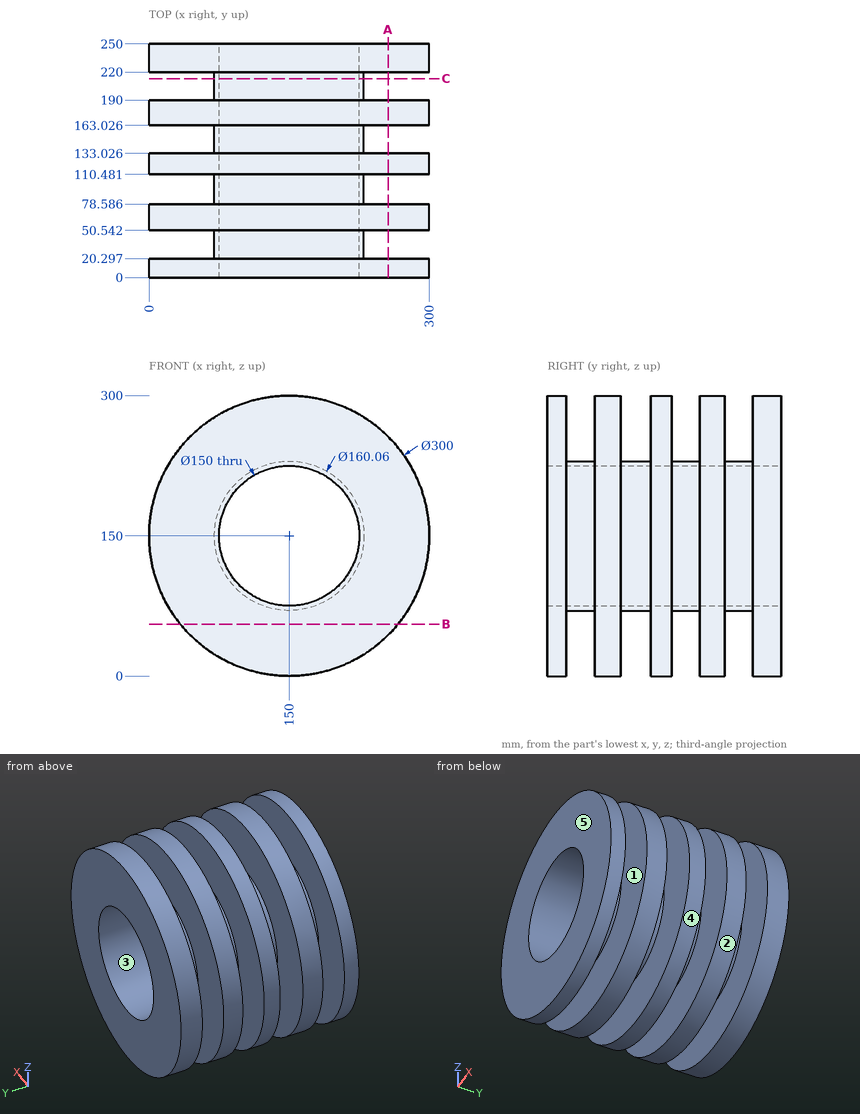
Source: three-view drawing plus pictorial views. Frame: mm from the lowest corner of the part. A direction names the side the tool comes from. Round coordinates to 2 decimals unless told otherwise and drop trailing zeros. Write each loop counter-clockwise with the first axis right and the second up, starting at its lowest first coordinate (ties: lowest second). Pieces come first, ordered by that corner, then holes. Notation, with made-up numbers: M 70,49.25 L 88,49.25 A6 cw 88,54.25 Z; hole C 71,54 d4. An arc over 180 degrees is marked long. One line per item, written item: value. Start each with the question number.
Item 1: Section query A-A (x = 256). Return the cut outline in (y, z).
Item 2: Section query C-C (y = 213). Return the cut outline in (x, z), plus the area to 3 significant figures.
Item 3: Set-up query: the marked faces 1 and 2. Return all of +Z, -Z, +X, -X, +Y, -Y with unobstructed straight access to the full face (end or side cutting, diameter ignored); none if empty.
Item 4: Mould query, pull axis Z, two halves, no side actions, for the marked faces 3, 4 and 5. Classes: pulls with the +Z half, pulls with the -Z half, needs draft (parallel to the pull), parting line crosses it, or undercut.
Item 5: Ray query, L1, parallel to Y at x = 188, z = 50; L2, parallel to X at y = 160.5, z = 150; L3, parallel to X at y = 62, z = 150. Return the intervals inside material, ascending. Write a range as from..to.
Item 6: Section query B-B (z = 55.5). Return the cut outline in (x, y).
Item 7: Pin query (flat end, axial travel): pin 1 (10 mm diameter, centred on y = 43.5, z = 195, fed in from -X); pin 2 (10 mm diameter, centred on y = 25, z = 208, fed in from +X); pin 3 (4 mm diameter, centred on y = 45, z = 214, fed in from -X) (1 decimal). Return the tip coordinate at first contact, or that it passes through.
Result set:
1. outline: M 0,43.87 L 20.3,43.87 L 20.3,256.13 L 0,256.13 Z; M 50.54,43.87 L 78.59,43.87 L 78.59,256.13 L 50.54,256.13 Z; M 110.48,43.87 L 133.03,43.87 L 133.03,256.13 L 110.48,256.13 Z; M 163.03,43.87 L 190,43.87 L 190,256.13 L 163.03,256.13 Z; M 220,43.87 L 250,43.87 L 250,256.13 L 220,256.13 Z
2. outline: C 150,150 d160.06; hole C 150,150 d150
2. area: 2,450 mm²
3. face 1: none
3. face 2: +Y, -Y
4. face 3: undercut
4. face 4: parting line crosses it
4. face 5: needs draft
5. L1: y = 0..20.3, 50.54..78.59, 110.48..133.03, 163.03..190, 220..250
5. L2: x = 69.97..75, 225..230.03
5. L3: x = 0..75, 225..300
6. outline: M 33.51,0 L 266.49,0 L 266.49,20.3 L 33.51,20.3 Z; M 33.51,50.54 L 266.49,50.54 L 266.49,78.59 L 33.51,78.59 Z; M 33.51,110.48 L 266.49,110.48 L 266.49,133.03 L 33.51,133.03 Z; M 33.51,163.03 L 266.49,163.03 L 266.49,190 L 33.51,190 Z; M 33.51,220 L 266.49,220 L 266.49,250 L 33.51,250 Z
7. pin 1: stops at x = 80.68
7. pin 2: stops at x = 289.03
7. pin 3: stops at x = 99.4
